Can you work these out from the model? Positions are in its coordinate system, mm. Coordinates: 2 decimals unless noted, no trailing zeros. Loops run counter-clockwise (first coordinate to the right, second up) from the corner with the lowest first, then second, coordinate; pieces in that order, holes last.
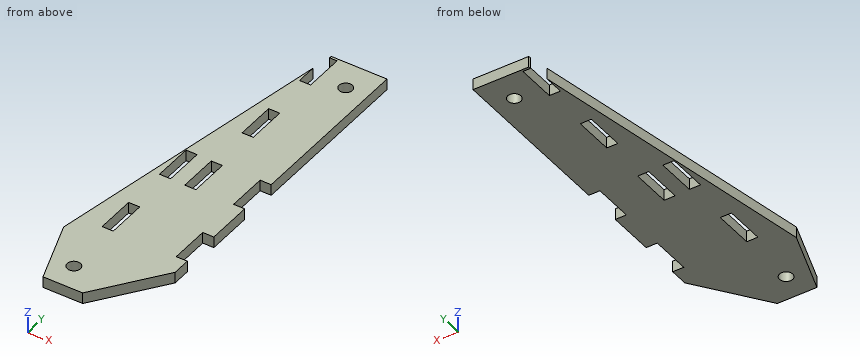
```python
from build123d import *

# Parameters (mm, degrees)
BODYSHAPE_DEPTH      = 5.334
SKETCH2_W            = 5.334
SKETCH2_H            = 19.05
MOTORMOUNTCUTS_DEPTH = 151.780754949
SKETCH3_R            = 3.175
BOLTHOLES_DEPTH      = 151.780754949
SKETCH4_W            = 5.334
SKETCH4_H            = 19.05
CUT_EXTRUDE3_DEPTH   = 151.780754949


with BuildPart() as part:
    # Sketch1 → BodyShape (new body)
    with BuildSketch(Plane.XY):
        Polygon((-80.812244673, 105.406062542), (-54.142244673, 105.406062542), (-54.142244673, -46.993937458), (-77.342244755, -78.743937458), (-96.392244755, -78.743937458), (-107.684476533, -46.993937458), align=None)
    extrude(amount=BODYSHAPE_DEPTH)

    # Sketch2 → MotorMountCuts (cut, through all)
    with BuildSketch(Plane.XY.offset(5.334)):
        with Locations((-56.809244673, -28.705937458)):
            Rectangle(SKETCH2_W, SKETCH2_H)
        with Locations((-56.809244673, 12.569062542)):
            Rectangle(SKETCH2_W, SKETCH2_H)
        with Locations((-92.369244673, -28.705937458)):
            Rectangle(SKETCH2_W, SKETCH2_H)
        with Locations((-92.369244673, 12.569062542)):
            Rectangle(SKETCH2_W, SKETCH2_H)
    extrude(amount=-MOTORMOUNTCUTS_DEPTH, mode=Mode.SUBTRACT)

    # Sketch3 → BoltHoles (cut, through all)
    with BuildSketch(Plane.XY.offset(5.334)):
        with Locations((-90.042244755, -66.043937458)):
            Circle(SKETCH3_R)
        with Locations((-64.642244755, 91.436062542)):
            Circle(SKETCH3_R)
    extrude(amount=-BOLTHOLES_DEPTH, mode=Mode.SUBTRACT)

    # Sketch4 → Cut-Extrude3 (cut, through all)
    with BuildSketch(Plane.XY.offset(5.334)):
        with Locations((-80.009244755, 94.771037838)):
            Rectangle(SKETCH4_W, SKETCH4_H)
        with Locations((-80.009244755, 53.496037838)):
            Rectangle(SKETCH4_W, SKETCH4_H)
        with Locations((-80.009244755, 12.221037838)):
            Rectangle(SKETCH4_W, SKETCH4_H)
    extrude(amount=-CUT_EXTRUDE3_DEPTH, mode=Mode.SUBTRACT)


solid = part.part
```
(1) I want a section at B-B on y = -33. Write out the boundary of the cut face in (x, z), then the cut area to 3 significant figures.
Check values:
outline: (-105.22, 0) - (-95.04, 0) - (-95.04, 5.33) - (-105.22, 5.33) - close; (-89.7, 0) - (-59.48, 0) - (-59.48, 5.33) - (-89.7, 5.33) - close
area: 216 mm2
(2) I want a section at A-A on x = -64.5. Write out the boundary of the cut face in (y, z), then the cut area to 3 significant figures.
Check values:
outline: (-61.17, 0) - (88.26, 0) - (88.26, 5.33) - (-61.17, 5.33) - close; (94.61, 0) - (105.41, 0) - (105.41, 5.33) - (94.61, 5.33) - close
area: 855 mm2
(3) I want a section at D-D on z = 3.3. State how many separate pieces and enclosed holes the cut face has, then the cut area to 3 significant figures.
Check values:
separate pieces: 1
enclosed holes: 6
area: 6,500 mm2
(4) If I drill on probe 1 along Y at (x, z) = (-80, 3); probe 2 along X at (y, z) = (17, 4.4); probe 3 along X at (y, z) = (18, 4.6), over which ranges is the centre line in solid material (lowest first)?
Check values:
probe 1: y = -78.74 to 2.7, 21.75 to 43.97, 63.02 to 85.25, 104.3 to 105.41
probe 2: x = -96.4 to -95.04, -89.7 to -82.68, -77.34 to -59.48
probe 3: x = -96.22 to -95.04, -89.7 to -82.68, -77.34 to -59.48
(5) I want a section at C-C on y = 15. Write out the boundary of the cut face in (x, z), then the cut area to 3 significant figures.
Check values:
outline: (-96.75, 0) - (-95.04, 0) - (-95.04, 5.33) - (-96.75, 5.33) - close; (-89.7, 0) - (-82.68, 0) - (-82.68, 5.33) - (-89.7, 5.33) - close; (-77.34, 0) - (-59.48, 0) - (-59.48, 5.33) - (-77.34, 5.33) - close
area: 142 mm2
(6) I'm going to push flat-ended pins straight in: pin 1 (2.5 mm diameter, centred on y = 8, z = 1.5, fed in from +X); pin 2 (1 mm diameter, centred on y = -34.5, z = 1, fed in from -X). Where does each tip first touch, or does it pass through?
Check values:
pin 1: stops at x = -59.48
pin 2: stops at x = -105.57
